Autodesk Inventor part; units mm, degrees
ref_plane "YZ Plane" through (0, 0, 0) normal (1, 0, 0) x (0, 1, 0)
ref_plane "XZ Plane" through (0, 0, 0) normal (0, 1, 0) x (-1, 0, 0)
ref_plane "XY Plane" through (0, 0, 0) normal (0, 0, 1) x (1, 0, 0)
sketch "Sketch1" plane through (0, 0, 0) normal (0, 0, 1) x (1, 0, 0)
  line L0 (0, 0) -> (24, 0)
  line L1 (24, 0) -> (24, 15.5)
  line L2 (24, 15.5) -> (0, 15.5)
  line L3 (0, 15.5) -> (0, 0)
  dimension "d0" = 24
  dimension "d1" = 15.5
extrude "Extrusion1" add sketch "Sketch1" along normal blind 5
sketch "Sketch7" plane through (0, 0, 5) normal (0, 0, 1) x (1, 0, 0)
  line L0 (24, 15.5) -> (0, 15.5)
  line L1 (0, 15.5) -> (0, 0)
  line L2 (5, 11.5) -> (19, 11.5)
  line L3 (19, 11.5) -> (19, 4)
  line L4 (19, 4) -> (5, 4)
  line L5 (5, 4) -> (5, 11.5)
  point P0 (12, 11.5)
  point P1 (12, 15.5)
  point P2 (5, 7.75)
  point P3 (0, 7.75)
  dimension "d21" = 14
  dimension "d22" = 7.5
extrude "Extrusion7" cut sketch "Sketch7" against normal blind 5
sketch "Sketch8" plane through (0, 0, 0) normal (0, -1, 0) x (1, 0, 0)
  line L0 (0, 0) -> (24, 0)
  line L1 (5, 5) -> (5, 0) construction
  line L2 (5, 5) -> (6, 5)
  line L3 (6, 5) -> (6, 0)
  line L4 (6, 0) -> (5, 0)
  line L5 (5, 0) -> (5, 5)
  line L6 (0, 0) -> (0, 5)
  dimension "d34" = 5
extrude "Extrusion8" cut sketch "Sketch8" against normal blind 5
sketch "Sketch9" plane through (0, 0, 5) normal (0, 0, 1) x (1, 0, 0)
  line L0 (6, 4) -> (6, 0)
  line L1 (6, 0) -> (24, 0)
  line L2 (24, 0) -> (24, 15.5)
  line L3 (24, 15.5) -> (0, 15.5)
  line L4 (0, 15.5) -> (0, 0)
  line L5 (0, 0) -> (5, 0)
  line L6 (5, 0) -> (5, 11.5)
  line L7 (5, 11.5) -> (19, 11.5)
  line L8 (19, 11.5) -> (19, 4)
  line L9 (19, 4) -> (6, 4)
extrude "Extrusion9" add sketch "Sketch9" along normal blind 2
sketch "Sketch10" plane through (0, 0, 0) normal (-1, 0, 0) x (0, 0, 1)
  circle A0 centre (3.5, 7.75) radius 2.15
  dimension "d30" = 4.3
extrude "Extrusion10" cut sketch "Sketch10" against normal blind 5
fillet "Fillet2" radius 2 4 edges at (24, 0, 3.5) (24, 15.5, 3.5) (0, 0, 3.5) (0, 15.5, 3.5)
properties part number "CounterWeightHook"
Check sheet for the modelled part. Datum: model origin and axes. Units: mm. A direction names the side the tool comes from. Round coordinates to 2 decimals unless told otherwise and drop trailing zeros. Loops run counter-clockwise (first coordinate to the right, second up) from the corner with the lowest first, then second, coordinate; pieces in that order, holes last. Notation, with made-up numbers: (-9.75, 14.25) - (8.25, 14.25) arc R29 ccw to (8.25, 45.25) - close; hole circle Ø3 at (63, 51.5). An arc over 180 degrees is marked (long way). Answer as a JSON object with one key per item and string values. Group by question number.
Q1. Mould release check, pull along X, two halves, no side actions. Record for faces 6 (the face through (23.4, 14.93, 3.45)), 7 (the face through (5, 4, 3)), 8 (the face through (0, 8, 1)), 9 (the face through (3, 0, 3)): released by +X, released by -X, zero draft, split by the parting line, or undercut.
Q2. Sectioned sample at A-A, the plane x = 10.25. Enter the section's corners in (y, z).
Q3. Scan lines: line 1 along Y through (x, z) = (13, 3); line 2 along Y through (x, z) = (3.9, 3.5); line 3 along X through (y, z) = (0.5, 5). Record each from-to range of solid material in increasing order. Write a range as [from, to].
Q4. Set-up check for faces 1 (the face through (0.57, 14.9, 3.45)), 2 (the face through (12, 3, 0)), 3 (the face through (6, 2, 3)), 4 (the face through (2.46, 9.88, 3.22)), 5 (the face through (12, 11.5, 3)): record each of +Z, -Z, +X, -X, +Y, -Y from which the full face is reachable in a straight line by a thin tool's end or side.
Q5. Sectioned sample at D-D, the plane z = 6.5. Enter the section's corners in (x, y), plus the area to 3 significant figures.
Q6. Sectioned sample at C-C, the plane z = 3.5. Enter the section's corners in (x, y).
Q7. Sectioned sample at B-B, the plane y = 7. Enter the section's corners in (x, z), plus the area to 3 significant figures.
Solution:
{
 "1": {"face 6": "released by +X", "face 7": "undercut", "face 8": "released by -X", "face 9": "zero draft"},
 "2": {"outline": "(0, 0) - (4, 0) - (4, 7) - (0, 7) - close; (11.5, 0) - (15.5, 0) - (15.5, 7) - (11.5, 7) - close"},
 "3": {"line 1": "y = [0, 4], [11.5, 15.5]", "line 2": "y = [0, 5.6], [9.9, 15.5]", "line 3": "x = [0.68, 5], [6, 23.32]"},
 "4": {"face 1": "+Z, -Z, -X, +Y", "face 2": "-Z, +X, -X, +Y, -Y", "face 3": "+Z, -Z, -Y", "face 4": "-X", "face 5": "+Z, -Z"},
 "5": {"outline": "(0, 2) arc R2 ccw to (2, 0) - (5, 0) - (5, 11.5) - (19, 11.5) - (19, 4) - (6, 4) - (6, 0) - (22, 0) arc R2 ccw to (24, 2) - (24, 13.5) arc R2 ccw to (22, 15.5) - (2, 15.5) arc R2 ccw to (0, 13.5) - close", "area": "260 mm²"},
 "6": {"outline": "(0, 2) arc R2 ccw to (2, 0) - (5, 0) - (5, 5.6) - (0, 5.6) - close; (0, 9.9) - (5, 9.9) - (5, 11.5) - (19, 11.5) - (19, 4) - (6, 4) - (6, 0) - (22, 0) arc R2 ccw to (24, 2) - (24, 13.5) arc R2 ccw to (22, 15.5) - (2, 15.5) arc R2 ccw to (0, 13.5) - close"},
 "7": {"outline": "(0, 0) - (5, 0) - (5, 1.49) - (0, 1.49) - close; (0, 5.51) - (5, 5.51) - (5, 7) - (0, 7) - close; (19, 0) - (24, 0) - (24, 7) - (19, 7) - close", "area": "49.9 mm²"}
}
